Read the model definition and answer for the solid it produces. Units are mm, in the model's axes. A direction names the side the tool comes from. Coordinates: 2 decimals unless noted, no trailing zeros. Write each loop counter-clockwise with the first axis right and the second up, starting at its lowest first coordinate (ties: lowest second). Pieces come first, ordered by that corner, then holes. Notation, with made-up numbers: (79.25, 15) -> (98.25, 15) arc R13 ccw to (98.25, 24) -> close; hole circle Ø7 at (18.5, -26.5). An arc over 180 degrees is marked (long way). Answer in a Markdown table with one row per item. Add a question column.
Item 1: Section C-C on z = 7.5 is taken. Write down the section's boundary in (x, y), then the cut area to 3 significant figures.
Item 2: Section D-D on x = -1.75 is taken. Write down the section's boundary in (y, z).
Item 3: Given pin 1 Ø4 at (y, z) = (10.5, 2.5) entering from +X; pin 2 Ø1 at (x, z) = (-1, 4.5) entering from -Y; pin 3 Ø1.5 at (y, z) = (2, 1.5) entering from -X; pin 4 Ø6 at (x, y) = (4, 16.5) entering from -Z, each flat-ended and moving along its own axis, determine where each tip first touches the part or whether it passes through.
Item 4: For a pull along Y with two mould halves and no side action, classify faces 1 (the face through (6.94, -1.03, 4.93)), 2 (the face through (8.5, 14.7, 0)), 3 (the face through (-9.566, 24.545, 5.07)) as +Y half, -Y half, draft (parallel to the pull), parting line (faces both ways), or undercut.
Item 5: Straight lines are drawn through the part: line 1 (X direction, y = 1.5, z = 6); line 2 (X direction, y = 6.75, z = 1.5); line 3 (Y direction, x = 2.5, z = 5.25). For each, find the intervals that lie inside material, in ascending order. Write a range as from..to.
Item 6: Section B-B on x = 7.75 is taken. Write down the section's boundary in (y, z).
Item 7: Which of the six approach directions +Z, -Z, +X, -X, +Y, -Y give full straight-line access (tool end or side, diameter ignored) to faces 4 (the face through (0, 27.393, 5)), 5 (the face through (-8.28, 15.14, 4.93))?
Item 8: Section A-A on y = 10.5 is taken. Write down the section's boundary in (x, z), then the cut area to 3 significant figures.
```python
from build123d import *

# Parameters (mm, degrees)
F1_DEPTH = 10
F2_R     = 1


with BuildPart() as f1:
    # F0 (on Top) → F1 (new body)
    with BuildSketch(Plane.XY):
        with BuildLine():
            Line((-10, 24.893011), (0, 24.893011))
            Line((0, 24.893011), (10, 24.893011))
            Line((10, 24.893011), (6.71487, 6.262112))
            ThreePointArc((6.71487, 6.262112), (3.462721, 1.577561), (6.71487, -3.106989))
            Line((6.71487, -3.106989), (7.001372, -0.450851))
            ThreePointArc((7.001372, -0.450851), (6.152804, 2.533741), (8.862567, 4.045379))
            Line((8.862567, 4.045379), (12.979384, 27.393011))
            Line((12.979384, 27.393011), (0, 27.393011))
            Line((0, 27.393011), (-12.979384, 27.393011))
            Line((-12.979384, 27.393011), (-8.862567, 4.045379))
            ThreePointArc((-8.862567, 4.045379), (-6.152804, 2.533741), (-7.001372, -0.450851))
            Line((-7.001372, -0.450851), (-6.71487, -3.106989))
            ThreePointArc((-6.71487, -3.106989), (-3.462721, 1.577561), (-6.71487, 6.262112))
            Line((-6.71487, 6.262112), (-10, 24.893011))
        make_face()
    extrude(amount=F1_DEPTH)

    # F2
    f2_edges = [f1.edges().sort_by_distance(p)[0] for p in [
        (-6.71487, -3.106989, 5),
        (6.71487, -3.106989, 5),
        (-12.979384, 27.393011, 5),
        (12.979384, 27.393011, 5),
        (-10, 24.893011, 5),
        (10, 24.893011, 5),
        (-6.71487, 6.262112, 5),
        (6.71487, 6.262112, 5),
        (-8.862567, 4.045379, 5),
        (8.862567, 4.045379, 5),
    ]]
    fillet(f2_edges, radius=F2_R)


solid = f1.part
```
Results below:
| question | item | result |
|---|---|---|
| 1 | outline | (-12.77, 26.22) -> (-9.01, 4.88) arc R1 ccw to (-8.15, 4.06) arc R2.5 cw to (-7, -0.45) -> (-6.88, -1.59) arc R1 ccw to (-5.24, -2.25) arc R5 ccw to (-6.26, 6.07) arc R1 cw to (-6.81, 6.79) -> (-9.79, 23.72) arc R1 cw to (-8.81, 24.89) -> (8.81, 24.89) arc R1 cw to (9.79, 23.72) -> (6.81, 6.79) arc R1 cw to (6.26, 6.07) arc R5 ccw to (5.24, -2.25) arc R1 ccw to (6.88, -1.59) -> (7, -0.45) arc R2.5 cw to (8.15, 4.06) arc R1 ccw to (9.01, 4.88) -> (12.77, 26.22) arc R1 ccw to (11.79, 27.39) -> (-11.79, 27.39) arc R1 ccw to start |
| 1 | area | 209 mm2 |
| 2 | outline | (24.89, 0) -> (27.39, 0) -> (27.39, 10) -> (24.89, 10) -> close |
| 3 | pin 1 | stops at x = 10.35 |
| 3 | pin 2 | stops at y = 24.89 |
| 3 | pin 3 | stops at x = -6.25 |
| 3 | pin 4 | passes through |
| 4 | face 1 | -Y half |
| 4 | face 2 | draft |
| 4 | face 3 | undercut |
| 5 | line 1 | x = -5.96..-3.46, 3.46..5.96 |
| 5 | line 2 | x = -9.34..-6.8, 6.8..9.34 |
| 5 | line 3 | y = 24.89..27.39 |
| 6 | outline | (3.97, 0) -> (12.13, 0) -> (12.13, 10) -> (3.97, 10) -> close; (24.89, 0) -> (27.39, 0) -> (27.39, 10) -> (24.89, 10) -> close |
| 7 | face 4 | +Z, -Z, +X, -X, +Y |
| 7 | face 5 | +Z, -Z |
| 8 | outline | (-10, 0) -> (-7.46, 0) -> (-7.46, 10) -> (-10, 10) -> close; (7.46, 0) -> (10, 0) -> (10, 10) -> (7.46, 10) -> close |
| 8 | area | 50.8 mm2 |
